Could you check a few things on this drawing? It's one solid part, dimensions in mm from its lowest x, y, z. Round coordinates to 2 decimals unless told otherwise and drop trailing zeros. Loops run counter-clockwise (first coordinate to the right, second up) from the corner with the lowest first, then second, coordinate; pieces in that order, holes last.
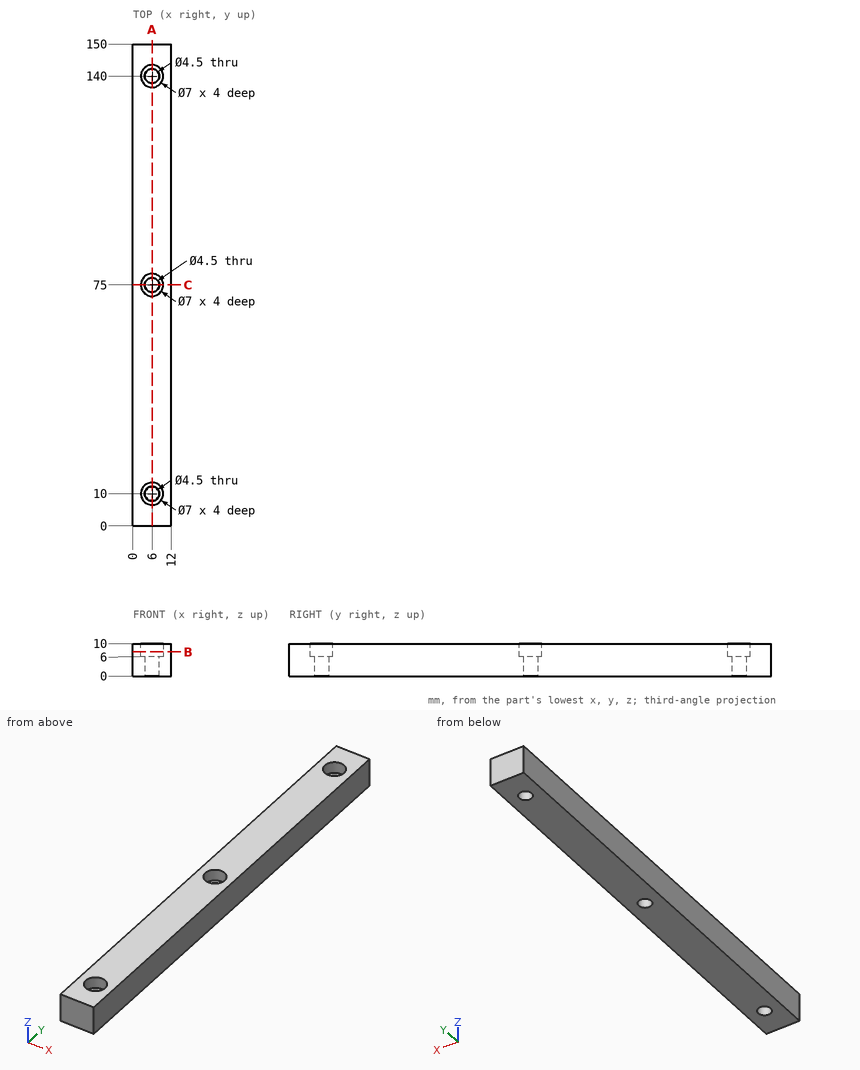
(1) For pin 1 (5.5 mm diameter, centred on x = 6, y = 75, fed in from +Z); pin 2 (4 mm diameter, centred on x = 6, y = 140, fed in from -Z), each with a flat end and sliding along its axis, tell me the tip position at first contact or that it passes through.
(2) Suppose I cut it at B-B (z = 7.5). Write out the boundary of the cut face in (x, y), then the cut area to 3 significant figures.
(3) Suppose I cut it at A-A (x = 6). Write out the boundary of the cut face in (y, z), then the cut area to 4 significant figures.
(4) If I drill on line 1 (Y direction, x = 6, z = 8.6); line 2 (Y direction, x = 6, z = 4.2); line 3 (X direction, y = 10, z = 3.7), over which ranges is the centre line in solid material (lowest first)?
(5) Suppose I cut it at C-C (y = 75). Write out the boundary of the cut face in (x, z).
Check result:
1. pin 1: stops at z = 6
1. pin 2: passes through
2. outline: (0, 0) - (12, 0) - (12, 150) - (0, 150) - close; hole circle Ø7 at (6, 10); hole circle Ø7 at (6, 75); hole circle Ø7 at (6, 140)
2. area: 1,680 mm2
3. outline: (0, 0) - (7.75, 0) - (7.75, 6) - (6.5, 6) - (6.5, 10) - (0, 10) - close; (12.25, 0) - (72.75, 0) - (72.75, 6) - (71.5, 6) - (71.5, 10) - (13.5, 10) - (13.5, 6) - (12.25, 6) - close; (77.25, 0) - (137.75, 0) - (137.75, 6) - (136.5, 6) - (136.5, 10) - (78.5, 10) - (78.5, 6) - (77.25, 6) - close; (142.25, 0) - (150, 0) - (150, 10) - (143.5, 10) - (143.5, 6) - (142.25, 6) - close
3. area: 1,335 mm2
4. line 1: y = 0 to 6.5, 13.5 to 71.5, 78.5 to 136.5, 143.5 to 150
4. line 2: y = 0 to 7.75, 12.25 to 72.75, 77.25 to 137.75, 142.25 to 150
4. line 3: x = 0 to 3.75, 8.25 to 12
5. outline: (0, 0) - (3.75, 0) - (3.75, 6) - (2.5, 6) - (2.5, 10) - (0, 10) - close; (8.25, 0) - (12, 0) - (12, 10) - (9.5, 10) - (9.5, 6) - (8.25, 6) - close
